Can you work these out from the drawing? Everything is in mm from the part's minimum corner. Coordinates: 2 decimals unless noted, no trailing zeros. Write each loop counter-clockwise with the first axis right and the second up, starting at its lowest first coordinate (ties: lowest second). Pieces come first, ordered by that corner, then holes.
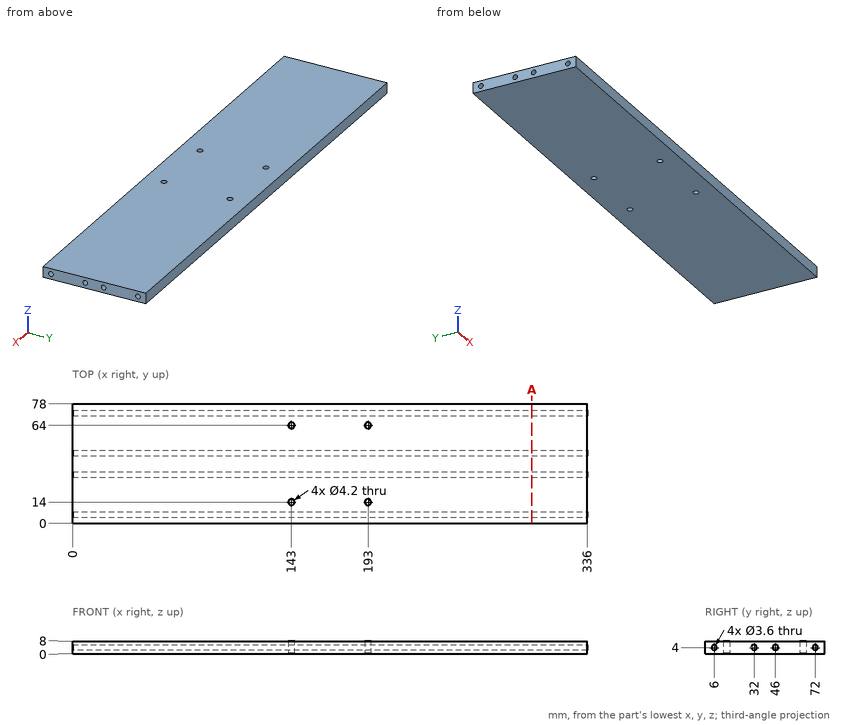
1. For pin 1 Ø3 at (y, z) = (32, 4) entering from -X, with a flat end and sliding along its axis, tell me the tip position at first contact or that it passes through.
2. I want a section at A-A (x = 300). List the corners of the cut face in (y, z) for me.
3. If I drill on line 1 (Y direction, x = 215.5, z = 4); line 2 (Y direction, x = 143, z = 6); line 3 (X direction, y = 64, z = 4.5), over which ranges is the centre line in solid material (lowest first)?
Response values:
1. pin 1: passes through
2. outline: (0, 0) - (78, 0) - (78, 8) - (0, 8) - close; hole circle Ø3.6 at (6, 4); hole circle Ø3.6 at (32, 4); hole circle Ø3.6 at (46, 4); hole circle Ø3.6 at (72, 4)
3. line 1: y = 0 to 4.2, 7.8 to 30.2, 33.8 to 44.2, 47.8 to 70.2, 73.8 to 78
3. line 2: y = 0 to 11.9, 16.1 to 61.9, 66.1 to 78
3. line 3: x = 0 to 140.9, 145.1 to 190.9, 195.1 to 336
